Geometry check sheet. Reference: the model listing, model coordinates, mm. A direction names the side the tool comes from. Coordinates: 2 decimals unless noted, no trailing zeros. Order: outer loops, then holes, each group sorted by start corner. A loop starts at its lowest first (then second) coordinate and runs counter-clockwise, first axis right, second up. Notation, with made-up numbers: (42, -30) - (61, -30) arc R20 cw to (61, -15) - close; hole circle Ø2 at (-10, 54). An arc over 180 degrees is marked (long way). One line per item, written item: value. Start each with the question number.
Autodesk Inventor part; units mm, degrees
ref_plane "YZ Plane" through (0, 0, 0) normal (1, 0, 0) x (0, 1, 0)
ref_plane "XZ Plane" through (0, 0, 0) normal (0, 1, 0) x (-1, 0, 0)
ref_plane "XY Plane" through (0, 0, 0) normal (0, 0, 1) x (1, 0, 0)
sketch "Sketch1" plane through (0, 0, 0) normal (0, 1, 0) x (-1, 0, 0)
  line L0 (-6.35, -6.35) -> (6.35, -6.35)
  line L1 (6.35, -6.35) -> (6.35, 6.35)
  line L2 (6.35, 6.35) -> (-6.35, 6.35)
  line L3 (-6.35, 6.35) -> (-6.35, -6.35)
  line L4 (-6.35, -6.35) -> (6.35, 6.35) construction
  line L5 (6.35, -6.35) -> (-6.35, 6.35) construction
  point P0 (0, 0)
  dimension "d0" = 12.7
  dimension "d1" = 12.7
extrude "Extrusion1" add sketch "Sketch1" along normal blind 1.5875
sketch "Sketch2" plane through (0, 1.5875, 0) normal (0, 1, 0) x (1, 0, 0)
  circle A0 centre (0, 0) radius 2.3812
  dimension "d4" = 4.7625
extrude "Extrusion2" cut sketch "Sketch2" against normal blind 1.5875
sketch "Sketch3" plane through (0, 1.5875, 0) normal (0, 1, 0) x (1, 0, 0)
  line L0 (-6.35, -6.35) -> (6.35, -6.35)
  line L1 (-6.35, -6.35) -> (6.35, -6.35)
  line L2 (6.35, -6.35) -> (6.35, -7.9375)
  line L3 (6.35, -7.9375) -> (-6.35, -7.9375)
  line L4 (-6.35, -7.9375) -> (-6.35, -6.35)
  line L5 (6.35, -6.35) -> (6.35, 6.35)
  line L6 (6.35, 6.35) -> (-6.35, 6.35)
  line L7 (-6.35, 6.35) -> (-6.35, 7.9375)
  line L8 (-6.35, 7.9375) -> (6.35, 7.9375)
  line L9 (6.35, 7.9375) -> (6.35, 6.35)
  point P0 (0, 0)
  dimension "d7" = 12.7
  dimension "d8" = 1.5875
  dimension "d9" = 12.7
  dimension "d10" = 1.5875
extrude "Extrusion3" add sketch "Sketch3" against normal blind 19.05
sketch "Sketch4" plane through (-6.35, 1.5875, 7.9375) normal (0, 0, 1) x (1, 0, 0)
  circle A0 centre (6.35, -12.7) radius 2.3813
  line L0 (12.7, 0) -> (12.7, -19.05)
  line L1 (12.7, -19.05) -> (0, -19.05)
  point P0 (6.35, -1.5875)
  dimension "d13" = 4.7625
  dimension "d14" = 6.35
  dimension "d15" = 6.35
extrude "Extrusion4" cut sketch "Sketch4" against normal blind 19.05
fillet "Fillet1" radius 1.5875 4 edges at (0, 1.5875, 7.9375) (0, 0, 6.35) (0, 0, -6.35) (0, 1.5875, -7.9375)
chamfer "Chamfer1" distance 1.5875 angle 45 4 edges at (6.35, -17.4625, 7.1437) (6.35, -17.4625, -7.1437) (-6.35, -17.4625, -7.1437) (-6.35, -17.4625, 7.1437)
properties part number "pnuematic bracket" material "Aluminum 6061"
Q1. Gauge pin test, flat ends, axial feed: P1, Ø2, axis at x = 0, z = 1, coming from the -Y side; P2, Ø7.5, axis at x = 2, z = -1.5, coming from the -Y side; P3, Ø1.5, axis at x = -2, z = 0.5, coming from the -Y side. Record the tip position at first contact, or that the pin passes through.
Q2. Release check for a two-part mould opening along Z. For faces 1 (the flat face through (-1.3, -8.6, 7.938)), 2 (the flat face through (6.35, 1, 0)), 3 (the flat face through (1.3, -8.6, -7.938)), 4 (the cylindrical face through (0.09, -0.45, 5.87)) record: released by +Z, released by -Z, zero draft, split by the parting line, or undercut.
Q3. Cross-section at C-C, the plane x = 0. Count the separate pieces of the cut face and the enclosed holes in it, and give its area (3 significant figures).
Q4. Cross-section at B-B, the plane z = 0. Enter the section's corners in (x, y).
Q5. Cross-section at D-D, the plane y = -9.5. Enter the section's corners in (x, z).
Q6. Material ranges on probe 1 along Z at (x, y) = (4.75, -10.5); probe 2 along Y at (x, z) = (2.75, -2.25); probe 3 along Y at (x, z) = (0, -7.55), recorded low to high.
Q7. Cross-section at A-A, the plane y = -6. Enter the section's corners in (x, z), and give its area (3 significant figures).
Q8. Set-up check for faces 5 (the flat face through (0, -17.462, -7)), 6 (the flat face through (-1.3, 0, 2.2)): record each of +Z, -Z, +X, -X, +Y, -Y from which the full face is reachable in a straight line by a thin tool's end or side.
Check result:
1. P1: passes through
1. P2: stops at y = -0.08
1. P3: stops at y = 0
2. face 1: released by +Z
2. face 2: zero draft
2. face 3: released by -Z
2. face 4: undercut
3. separate pieces: 4
3. enclosed holes: 0
3. area: 58.0 mm2
4. outline: (-6.35, 0) - (-2.38, 0) - (-2.38, 1.59) - (-6.35, 1.59) - close; (2.38, 0) - (6.35, 0) - (6.35, 1.59) - (2.38, 1.59) - close
5. outline: (-6.35, -7.94) - (-1.75, -7.94) - (-1.75, -6.35) - (-6.35, -6.35) - close; (-6.35, 6.35) - (-1.75, 6.35) - (-1.75, 7.94) - (-6.35, 7.94) - close; (1.75, -7.94) - (6.35, -7.94) - (6.35, -6.35) - (1.75, -6.35) - close; (1.75, 6.35) - (6.35, 6.35) - (6.35, 7.94) - (1.75, 7.94) - close
6. probe 1: z = -7.94 to -6.35, 6.35 to 7.94
6. probe 2: y = 0 to 1.59
6. probe 3: y = -17.46 to -13.49, -8.73 to 1.04
7. outline: (-6.35, -7.94) - (6.35, -7.94) - (6.35, -6.35) - (-6.35, -6.35) - close; (-6.35, 6.35) - (6.35, 6.35) - (6.35, 7.94) - (-6.35, 7.94) - close
7. area: 40.3 mm2
8. face 5: +Z, -Z, +X, -X, -Y
8. face 6: +X, -X, -Y
